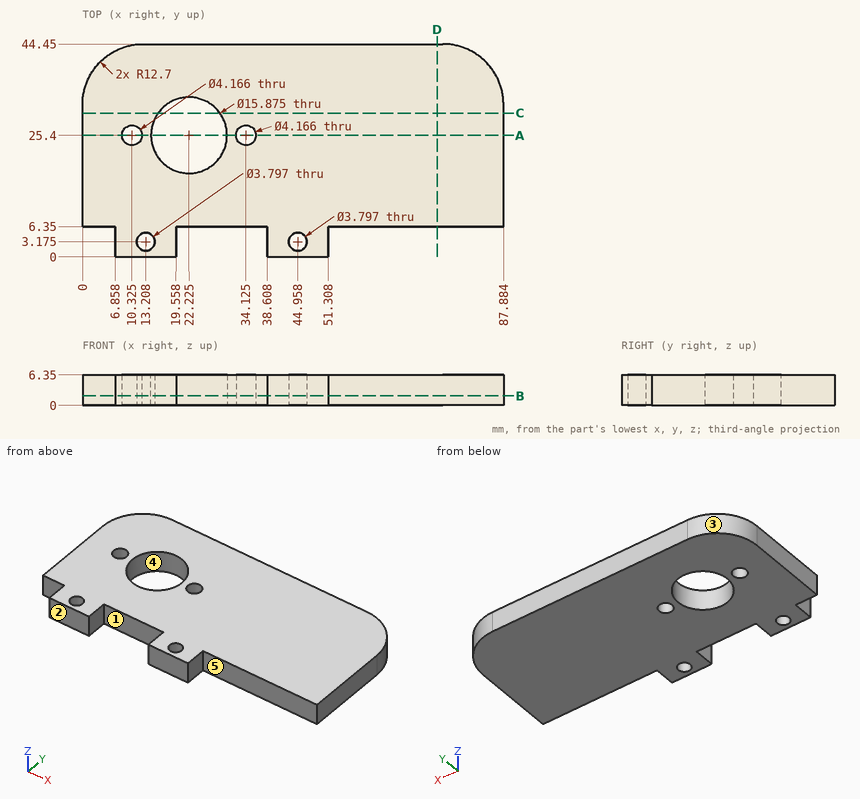
Geometry check sheet. Reference: drawing and pictorial views, mm from the part's lowest x, y, z. A direction names the side the tool comes from. Give positions to 0.01 mm unless a question says otherwise; leave off trailing zeros. Write each loop counter-clockwise with the first axis right and the second up, starting at its lowest first coordinate (ties: lowest second). Pieces come first, ordered by that corner, then holes. Notation, with made-up numbers: M -29,-4.5 L 25,-4.5 A10 ccw 25,14.5 Z; hole C 7.5,-36.75 d4. An arc over 180 degrees is marked long. Answer as CSV lines item,"result". Start each with the question number.
Q1. Tool access check on the marked faces 1 and 2. Record the directions out of +Z, -Z, +X, -X, +Y, -Y that give a thin tool (end or side, any length) a straight path to the whole face; none if there is none.
Q2. Release check for a two-part mould opening along X. For the marked faces 3, 4 and 5 record: pulls with the +X half, pulls with the -X half, needs draft (parallel to the pull), parting line crosses it, or undercut.
Q3. Section check A-A, the plane y = 25.4. Record the cut outline in (x, z), then the cut area to 3 significant figures.
Q4. Material ranges on L1, parallel to X at y = 25.5, z = 2.25 (1 decimal); L2, parallel to X at y = 4.5, z = 3.5; L3, parallel to X at y = 6, z = 3.5, recorded low to high.
Q5. Section check C-C, the plane y = 30. Record the cut outline in (x, z).
Q6. Go/stop test with flat-tipped pins: pin 1 (3.5 mm diameter, centred on x = 44.958, y = 3.175, fed in from +Z); pin 2 (1 mm diameter, centred on x = 9, z = 5, fed in from +Y); pin 3 (5.5 mm diameter, centred on x = 34.12, y = 25.4, fed in from -Z); pin 4 (1.9 mm diameter, centred on x = 70.5, z = 2, fed in from -Y). Record where each tip stops, or that it passes through.
Q7. Section check B-B, the plane z = 2. Give the number of separate pieces and of enclosed holes in the cut face, then the cut area to 3 significant figures.
Q8. Section check D-D, the plane x = 74. Record the cut outline in (y, z).
Geometry says:
1,face 1,"+Z, -Z, -Y"
1,face 2,"+Z, -Z, +X, -X, -Y"
2,face 3,"pulls with the -X half"
2,face 4,"undercut"
2,face 5,"needs draft"
3,outline,"M 0,0 L 8.24,0 L 8.24,6.35 L 0,6.35 Z; M 12.41,0 L 14.29,0 L 14.29,6.35 L 12.41,6.35 Z; M 30.16,0 L 32.04,0 L 32.04,6.35 L 30.16,6.35 Z; M 36.21,0 L 87.88,0 L 87.88,6.35 L 36.21,6.35 Z"
3,area,"404 mm^2"
4,L1,"0 to 8.2, 12.4 to 14.3, 30.2 to 32, 36.2 to 87.9"
4,L2,"6.86 to 11.85, 14.57 to 19.56, 38.61 to 43.6, 46.32 to 51.31"
4,L3,"6.86 to 19.56, 38.61 to 51.31"
5,outline,"M 0,0 L 15.76,0 L 15.76,6.35 L 0,6.35 Z; M 28.69,0 L 87.88,0 L 87.88,6.35 L 28.69,6.35 Z"
6,pin 1,"through"
6,pin 2,"y = 44.04"
6,pin 3,"z = 0"
6,pin 4,"y = 6.35"
7,separate pieces,"1"
7,enclosed holes,"5"
7,area,"3,190 mm^2"
8,outline,"M 6.35,0 L 44.45,0 L 44.45,6.35 L 6.35,6.35 Z"
